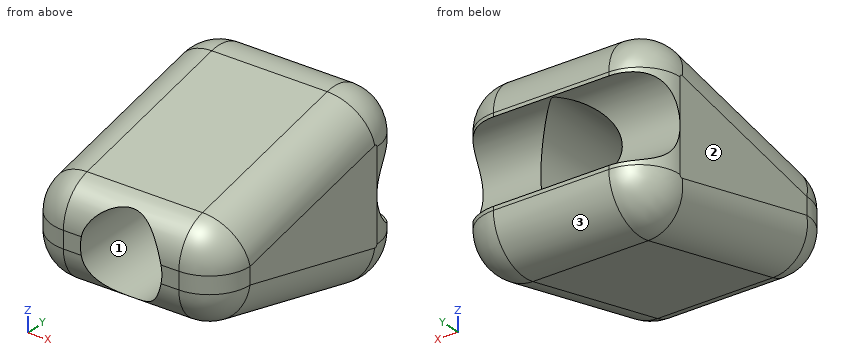
from build123d import *

# Parameters (mm, degrees)
F2_DEPTH = 14.5
F4_DEPTH = 29.001
F5_R     = 5.99999
F0_R     = 6
F6_DEPTH = 87.122


# Not quite as in the source:
# - a fillet or chamfer is up to 0.001 mm smaller than in the source, because OpenCascade refuses the exact size


with BuildPart() as f2:
    # F1 (on Right) → F2 (new body, symmetric)
    with BuildSketch(Plane.YZ):
        with BuildLine():
            Line((29.2391964545, 12.7315542681), (0, 6.0688508675))
            Line((0, 6.0688508675), (0, -5.9945774265))
            Line((0, -5.9945774265), (29.2273893105, -12.7132611239))
            ThreePointArc((29.2273893105, -12.7132611239), (34.6053079603, -11.4923680491), (37, -6.524668487))
            Line((37, -6.524668487), (37, 6.5402593021))
            ThreePointArc((37, 6.5402593021), (34.610044033, 11.5041842871), (29.2391964545, 12.7315542681))
        make_face()
    extrude(amount=F2_DEPTH, both=True)

    # F3 (on face) → F4 (cut, through all)
    with BuildSketch(Plane.YZ.offset(14.5)):
        with BuildLine():
            Line((37, -5.9922045925), (37, 6.0077954075))
            ThreePointArc((37, 6.0077954075), (31, 0.0077954075), (37, -5.9922045925))
        make_face()
    extrude(amount=-F4_DEPTH, mode=Mode.SUBTRACT)

    # F5 (radius 6 in the source; OpenCascade refuses exactly that, so slightly less here)
    f5_edges = [f2.edges().sort_by_distance(p)[0] for p in [
        (14.5, 14.619598, 9.400203),
        (14.5, 14.613695, -9.353919),
        (0, 37, 6.540259),
        (-14.5, 14.619598, 9.400203),
        (-14.5, 14.613695, -9.353919),
        (0, 0, -5.994577),
        (0, 0, 6.068851),
        (14.5, 0, 0.037137),
        (-14.5, 0, 0.037137),
    ]]
    fillet(f5_edges, radius=F5_R)

    # F0 (on Front) → F6 (cut)
    with BuildSketch(Plane.XZ):
        Circle(F0_R)
    extrude(amount=-F6_DEPTH, mode=Mode.SUBTRACT)


solid = f2.part
Read the model definition and answer for the solid it produces. Units are mm, in the model's axes. Face numbers are marked on the shaded views. Coordinates: 2 decimals unless noted, no trailing zeros. Loops run counter-clockwise (first coordinate to the right, second up) from the corner with the lowest first, then second, coordinate; pieces in that order, holes last. Notation, with made-up numbers: (-38.75, 84) -> (-11.75, 84) arc R28 cw to (-11.75, 123) -> close; hole circle Ø10 at (49.5, -33.75). An arc over 180 degrees is marked (long way). Answer in a Markdown table with one row per item.
Item 1: Straight lines are drawn through the part: line 1 along X through (y, z) = (18, 0); line 2 along Z through (x, y) = (0, 18); line 3 along Z through (x, y) = (0, 26). For each, find the intervals that lie inside material, in ascending order. Write a range as [from, to].
Returned:
| item | result |
|---|---|
| line 1 | x = [-14.5, -6], [6, 14.5] |
| line 2 | z = [-10.13, -6], [6, 10.17] |
| line 3 | z = [-11.97, -6], [6, 11.99] |
Item 2: Each of these flat-tipped pins is pushed along its axis until it touches: P1, Ø12, axis at x = -8.5, z = -8, coming from the -Y side; P2, Ø2, axis at x = -6, z = 6.5, coming from the -Y side; P3, Ø1, axis at x = -11.5, z = -2, coming from the -Y side. Where does it stop, or does it pass through?
Returned:
| item | result |
|---|---|
| P1 | stops at y = 0.05 |
| P2 | stops at y = 1.73 |
| P3 | stops at y = 0.59 |
Item 3: A cutting plane is placed at A-A on x = -6.75. Determine the outline of the cut face in (y, z), plus the area to 3 significant figures.
Returned:
| item | result |
|---|---|
| outline | (0, -1.22) arc R6 ccw to (4.66, -7.06) -> (29.23, -12.71) arc R6.35 ccw to (37, -6.52) -> (37, -5.99) arc R6 cw to (37, 6.01) -> (37, 6.54) arc R6.35 ccw to (29.24, 12.73) -> (4.67, 7.13) arc R6 ccw to (0, 1.28) -> close |
| area | 665 mm^2 |
Item 4: For a pull along Z with two mould halves and no side action, classify the marked faces 1, 2 and 3 as released by +Z, released by -Z, zero draft, split by the parting line, or undercut.
Returned:
| item | result |
|---|---|
| face 1 | undercut |
| face 2 | zero draft |
| face 3 | released by -Z |
Item 5: A cutting plane is placed at B-B on x = 3. Determine the outline of the cut face in (y, z), plus the area to 3 significant figures.
Returned:
| item | result |
|---|---|
| outline | (1.45, 5.2) -> (33.99, 5.2) arc R6 cw to (37, 6.01) -> (37, 6.54) arc R6.35 ccw to (29.24, 12.73) -> (4.67, 7.13) arc R6 ccw to start; (1.51, -5.2) arc R6 ccw to (4.66, -7.06) -> (29.23, -12.71) arc R6.35 ccw to (37, -6.52) -> (37, -5.99) arc R6 cw to (34.01, -5.2) -> close |
| area | 338 mm^2 |
